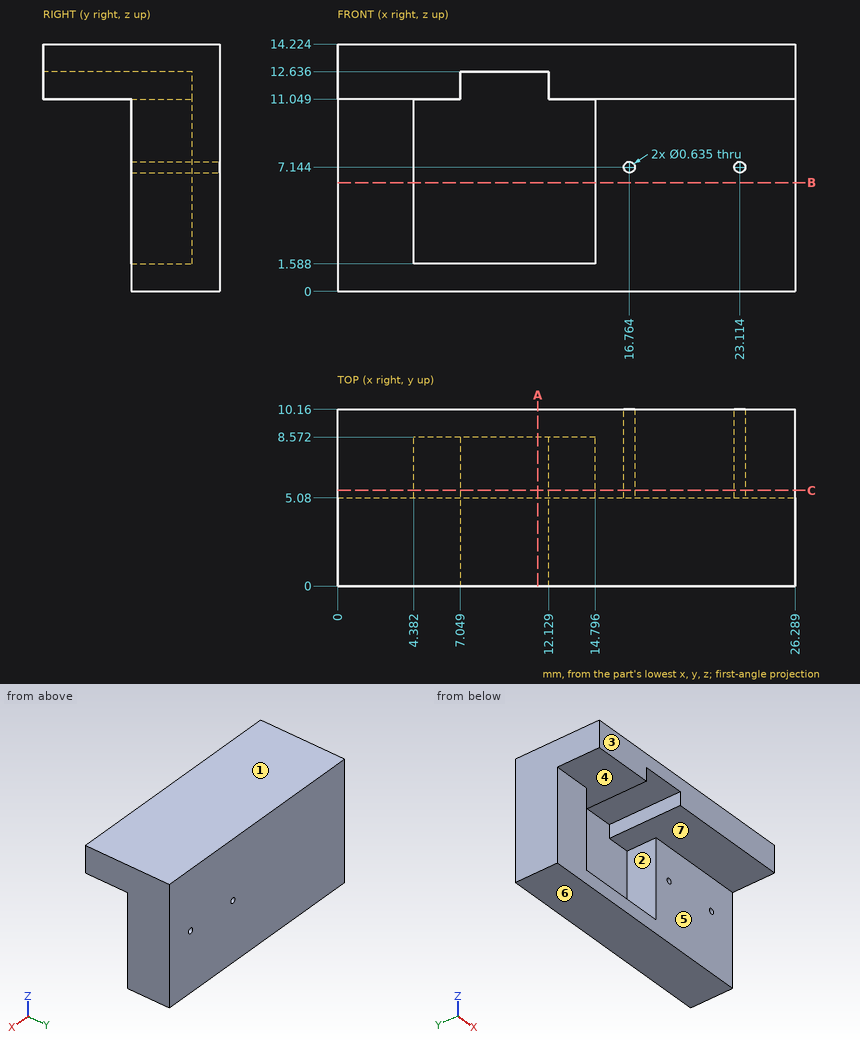
Study the drawing (mm; zero at the part's minimum x, y, z) and answer. A direction names the side the tool comes from. Give positions to 0.01 mm unless a question says otherwise; leave off trailing zeros. Loops run counter-clockwise (first coordinate to the right, second up) from the corner with the lowest first, then second, coordinate; pieces in that order, holes last. Notation, with made-up numbers: M -29,-37 L -6,-37 A15 cw -6,-28 Z; hole C 57,75 d3. An arc over 180 degrees is marked long. Use CSV: the item, a comma, the result in double quotes.
1) Find section A-A on x = 11.5. Write down the section's boundary in (y, z) (1 decimal).
Answer:
outline,"M 0,12.6 L 8.6,12.6 L 8.6,1.6 L 5.1,1.6 L 5.1,0 L 10.2,0 L 10.2,14.2 L 0,14.2 Z"
2) Find section B-B on z = 6.25. Write down the section's boundary in (x, y) (1 decimal).
Answer:
outline,"M 0,5.1 L 4.4,5.1 L 4.4,8.6 L 14.8,8.6 L 14.8,5.1 L 26.3,5.1 L 26.3,10.2 L 0,10.2 Z"
3) Given P1, Ø8.5, axis at x = 8.5, z = 6.5, coming from the -Y side; P2, Ø4, axis at x = 6, y = 2, coming from the -Z side; P3, Ø1, axis at x = 8, z = 4.5, coming from the -Y side, each flat-ended and moving along its own axis, determine where each tip first touches the part or whether it passes through.
Answer:
P1,"y = 5.08"
P2,"z = 11.05"
P3,"y = 8.57"
4) Find section C-C on y = 5.5. Give the number of separate pieces and of enclosed holes in the cut face, plus the area to 3 significant figures.
Answer:
separate pieces,"1"
enclosed holes,"3"
area,"267 mm^2"
5) Which of the six approach directions +Z, -Z, +X, -X, +Y, -Y give full straight-line access (tool end or side, diameter ignored) to the marked faces 5, 6 and 7?
Answer:
face 5,"-Z, +X, -X, -Y"
face 6,"-Z, +X, -X, +Y, -Y"
face 7,"-Y"
6) Consider L1, parallel to X at y = 5, z = 11.75; L2, parallel to Z at x = 8, y = 6 (1 decimal); L3, parallel to X at y = 5.5, z = 10.5 (1 decimal). Determine where each line is inside the solid, lowest interval first.
Answer:
L1,"0 to 7.05, 12.13 to 26.29"
L2,"0 to 1.6, 12.6 to 14.2"
L3,"0 to 4.4, 14.8 to 26.3"
7) Determine the mould class of the marked faces 1, 2, 3 and 4 for opening direction Z: released by +Z, released by -Z, zero draft, split by the parting line, or undercut.
Answer:
face 1,"released by +Z"
face 2,"undercut"
face 3,"zero draft"
face 4,"undercut"
